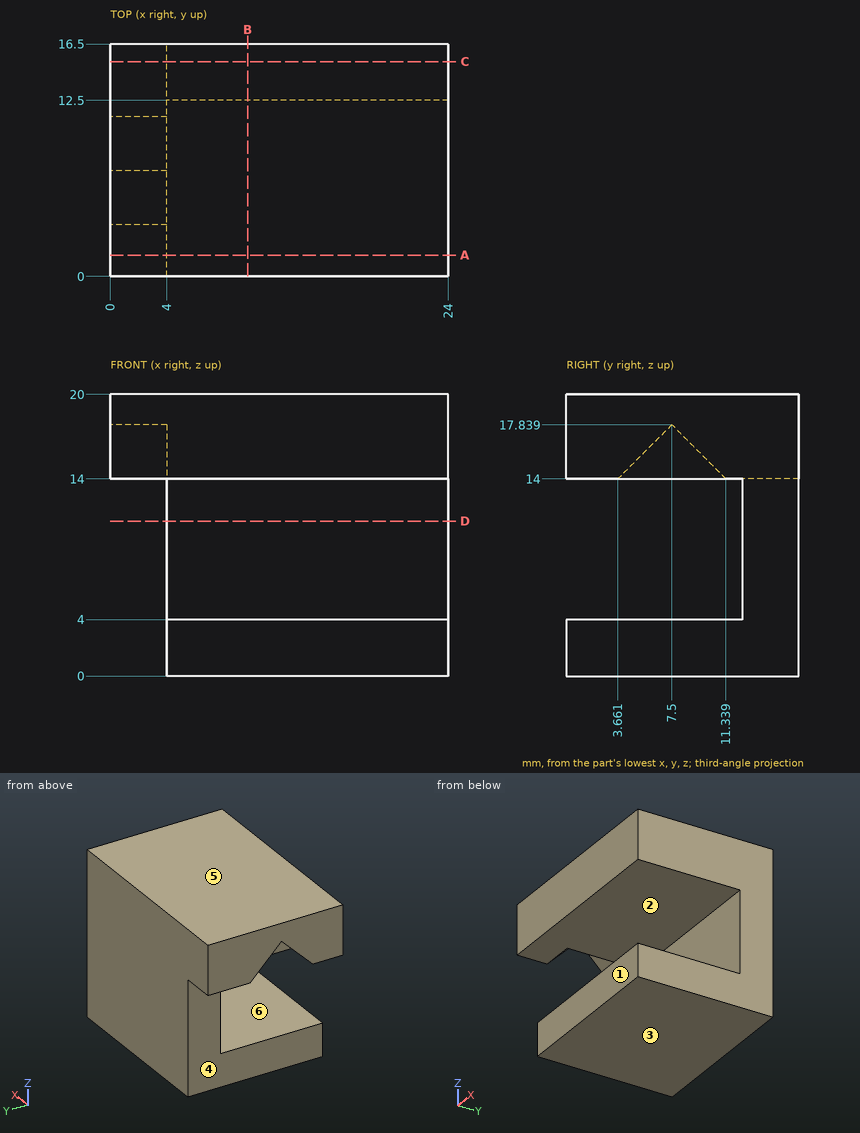
Can you work these out from the drawing? Everything is in mm from the part's minimum corner. A direction names the side the tool comes from. Coordinates: 2 decimals unless noted, no trailing zeros. Loops run counter-clockwise (first coordinate to the right, second up) from the corner with the lowest first, then second, coordinate; pieces in that order, holes last.
1) Imagine slicing it at A-A (y = 1.5). List the corners of the cut face in (x, z) for me.
Reported:
outline: (0, 14) - (24, 14) - (24, 20) - (0, 20) - close; (4, 0) - (24, 0) - (24, 4) - (4, 4) - close
2) Imagine slicing it at C-C (y = 15.25). List the corners of the cut face in (x, z) for me.
Reported:
outline: (0, 14) - (4, 14) - (4, 0) - (24, 0) - (24, 20) - (0, 20) - close
3) Imagine slicing it at B-B (x = 9.75). List the corners of the cut face in (y, z) for me.
Reported:
outline: (0, 0) - (16.5, 0) - (16.5, 20) - (0, 20) - (0, 14) - (12.5, 14) - (12.5, 4) - (0, 4) - close
4) Thinking about a two-plate mould opening in Z: for the marked faces 1, 2 and 3, which applies, released by +Z, released by -Z, zero draft, split by the parting line, or undercut?
Reported:
face 1: zero draft
face 2: undercut
face 3: released by -Z
5) Imagine slicing it at D-D (z = 11). List the corners of the cut face in (x, y) for me, and give its area (3 significant figures).
Reported:
outline: (4, 12.5) - (24, 12.5) - (24, 16.5) - (4, 16.5) - close
area: 80.0 mm2
6) Which directions (+Z, -Z, +X, -X, +Y, -Y) give clear straight access to the entire face, cutting with the end or side of a thin tool? Please do the marked faces 4, 5 and 6.
Reported:
face 4: -Z, -X, +Y, -Y
face 5: +Z, +X, -X, +Y, -Y
face 6: +X, -X, -Y
7) Please list where these lines run through material, in increasing order: line 1 along Z through (x, y) = (19.75, 2); line 2 along X through (y, z) = (15, 9.5); line 3 along Y through (x, z) = (20.5, 11).
Reported:
line 1: z = 0 to 4, 14 to 20
line 2: x = 4 to 24
line 3: y = 12.5 to 16.5
